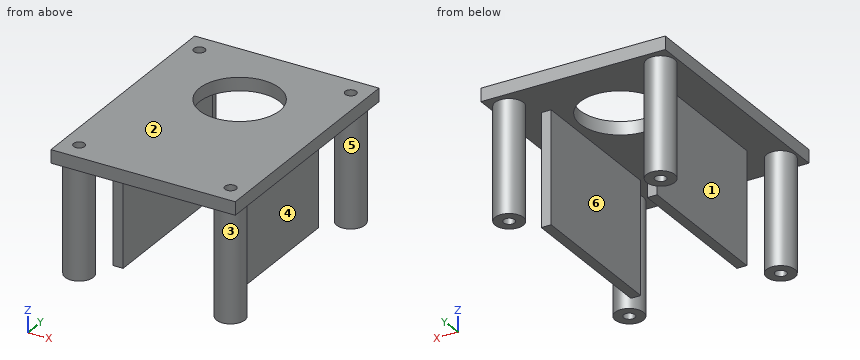
Solid Edge part; units mm, degrees
sketch "Sketch1" plane through (0, 0, -2.2) normal (0, 0, 1) x (1, 0, 0)
  line L0 (-28, -49) -> (28, -49)
  line L1 (28, -49) -> (28, 24)
  line L2 (28, 24) -> (-28, 24)
  line L3 (-28, 24) -> (-28, -49)
  circle A0 centre (0, 0) radius 12.2
  circle A1 centre (-23, -43) radius 1.7
  circle A2 centre (23, -43) radius 1.7
  circle A3 centre (-23, 18) radius 1.7
  circle A4 centre (23, 18) radius 1.7
extrude "ExtrudedProtrusion_1" add sketch "Sketch1" along normal blind 4
sketch "Sketch2" plane through (0, 0, -36.2) normal (0, 0, 1) x (1, 0, 0)
  circle A0 centre (-23, -43) radius 4.3
  circle A1 centre (-23, -43) radius 1.7
extrude "ExtrudedProtrusion_2" add sketch "Sketch2" along normal blind 34
sketch "Sketch3" plane through (0, 0, -36.2) normal (0, 0, 1) x (1, 0, 0)
  circle A0 centre (23, -43) radius 4.3
  circle A1 centre (23, -43) radius 1.7
extrude "ExtrudedProtrusion_3" add sketch "Sketch3" along normal blind 34
sketch "Sketch4" plane through (0, 0, -36.2) normal (0, 0, 1) x (1, 0, 0)
  circle A0 centre (-23, 18) radius 4.3
  circle A1 centre (-23, 18) radius 1.7
extrude "ExtrudedProtrusion_4" add sketch "Sketch4" along normal blind 34
sketch "Sketch5" plane through (0, 0, -36.2) normal (0, 0, 1) x (1, 0, 0)
  circle A0 centre (23, 18) radius 4.3
  circle A1 centre (23, 18) radius 1.7
extrude "ExtrudedProtrusion_5" add sketch "Sketch5" along normal blind 34
sketch "Sketch6" plane through (0, 0, -36.2) normal (0, 0, 1) x (1, 0, 0)
  line L0 (-17.6, -34.75) -> (-14.6, -34.75)
  line L1 (-14.6, -34.75) -> (-14.6, 10.75)
  line L2 (-14.6, 10.75) -> (-17.6, 10.75)
  line L3 (-17.6, 10.75) -> (-17.6, -34.75)
extrude "ExtrudedProtrusion_6" add sketch "Sketch6" along normal blind 34
sketch "Sketch7" plane through (0, 0, -36.2) normal (0, 0, 1) x (1, 0, 0)
  line L0 (14.6, -34.75) -> (17.6, -34.75)
  line L1 (17.6, -34.75) -> (17.6, 10.75)
  line L2 (17.6, 10.75) -> (14.6, 10.75)
  line L3 (14.6, 10.75) -> (14.6, -34.75)
extrude "ExtrudedProtrusion_7" add sketch "Sketch7" along normal blind 34
For this review, take the finished solid that the model builds, in its own axes (mm). Face numbers are marked on the shaded views. A direction names the side the tool comes from. Round coordinates to 2 decimals unless told otherwise and drop trailing zeros. Write each loop counter-clockwise with the first axis right and the second up, starting at its lowest first coordinate (ties: lowest second). Pieces come first, ordered by that corner, then holes.
1) Mouldability with a two-part tool opening along X and no side actions: class the marked faces 1, 2 and 3 as +X half, -X half, draft (parallel to the pull), parting line (faces both ways), or undercut.
Answer below:
face 1: -X half
face 2: draft
face 3: undercut
2) Take a section at D-D on y = 0. Give the boundary of the cut face in (x, z).
Answer below:
outline: (-28, -2.2) - (-17.6, -2.2) - (-17.6, -36.2) - (-14.6, -36.2) - (-14.6, -2.2) - (-12.2, -2.2) - (-12.2, 1.8) - (-28, 1.8) - close; (12.2, -2.2) - (14.6, -2.2) - (14.6, -36.2) - (17.6, -36.2) - (17.6, -2.2) - (28, -2.2) - (28, 1.8) - (12.2, 1.8) - close
3) Take a section at B-B on y = -43. Give the boundary of the cut face in (x, z).
Answer below:
outline: (-28, -2.2) - (-27.3, -2.2) - (-27.3, -36.2) - (-24.7, -36.2) - (-24.7, 1.8) - (-28, 1.8) - close; (-21.3, -36.2) - (-18.7, -36.2) - (-18.7, -2.2) - (18.7, -2.2) - (18.7, -36.2) - (21.3, -36.2) - (21.3, 1.8) - (-21.3, 1.8) - close; (24.7, -36.2) - (27.3, -36.2) - (27.3, -2.2) - (28, -2.2) - (28, 1.8) - (24.7, 1.8) - close
4) For line 1 along Y through (x, z) = (23, -18); line 2 along X through (y, z) = (-17, -30); line 3 along Y through (x, z) = (24.5, 0), list the stretches that pass through material, from the lowest coordinate up.
Answer below:
line 1: y = -47.3 to -44.7, -41.3 to -38.7, 13.7 to 16.3, 19.7 to 22.3
line 2: x = -17.6 to -14.6, 14.6 to 17.6
line 3: y = -49 to -43.8, -42.2 to 17.2, 18.8 to 24
5) Insertion check: pin 1 Ø17 at (x, y) = (-13, -19) entering from -Z; pin 2 Ø4 at (y, z) = (-37.5, -25.5) entering from +X; pin 3 Ø8 at (x, z) = (-13, -30) entering from +Y; pin 4 Ø1.5 at (x, y) = (-3.5, -38) entering from -Z. Each pin has a flat end and moves straight along its axis. Give the tip position at first contact, or say it passes through.
Answer below:
pin 1: stops at z = -36.2
pin 2: stops at x = 25.5
pin 3: stops at y = 10.75
pin 4: stops at z = -2.2
6) Take a section at C-C on x = 0. Give the boundary of the cut face in (y, z).
Answer below:
outline: (-49, -2.2) - (-12.2, -2.2) - (-12.2, 1.8) - (-49, 1.8) - close; (12.2, -2.2) - (24, -2.2) - (24, 1.8) - (12.2, 1.8) - close
7) Machinability: for the marked faces 4, 5 and 6, which of the approach directions +Z, -Z, +X, -X, +Y, -Y give a long, thin tool a straight path to every point of the face, cutting with its end or side? Answer none if there is none.
Answer below:
face 4: -Z, +X, +Y, -Y
face 5: -Z
face 6: -Z, +Y, -Y
8) Take a section at A-A on z = -12.5. State how many separate pieces and enclosed holes the cut face has, then the cut area to 3 significant figures.
Answer below:
separate pieces: 6
enclosed holes: 4
area: 469 mm2
